```python
from build123d import *

# Parameters (mm, degrees)
PAD_DEPTH         = 18
PAD001_DEPTH      = 5
SKETCH002_W       = 13.704409
SKETCH002_H       = 6
POCKET_DEPTH      = 10.001
POCKET_DEPTH_BACK = -10.001
SKETCH003_R       = 6
PAD002_DEPTH      = 10
SKETCH004_R       = 1.5
POCKET001_DEPTH   = 10


with BuildPart() as part:
    # Sketch → Pad (new body)
    with BuildSketch(Plane.XY):
        with BuildLine():
            Line((-10, 0), (10, 0))
            Line((10, 0), (10, 8))
            Line((10, 8), (3.527972, 11.180071))
            ThreePointArc((3.527972, 11.180071), (0, 12), (-3.527972, 11.180071))
            Line((-3.527972, 11.180071), (-10, 8))
            Line((-10, 8), (-10, 0))
        make_face()
    extrude(amount=PAD_DEPTH)

    # Sketch001 → Pad001 (join)
    with BuildSketch(Plane.XY):
        with BuildLine():
            Line((-10, 0), (10, 0))
            Line((10, 0), (10, 10))
            ThreePointArc((10, 10), (0, 20), (-10, 10))
            Line((-10, 10), (-10, 0))
        make_face()
    extrude(amount=PAD001_DEPTH)

    # Sketch002 → Pocket (cut, two sides)
    with BuildSketch(Plane.YZ) as pocket_sk:
        with Locations((11.852204, 8)):
            Rectangle(SKETCH002_W, SKETCH002_H)
    extrude(amount=-POCKET_DEPTH, mode=Mode.SUBTRACT)
    extrude(pocket_sk.sketch, amount=-POCKET_DEPTH_BACK, mode=Mode.SUBTRACT)

    # Sketch003 (on Face4 of Pocket) → Pad002 (join)
    with BuildSketch(Plane(origin=(0, 0, 0), x_dir=(1, 0, 0), z_dir=(0, 0, -1))):
        with Locations((0, -10)):
            Circle(SKETCH003_R)
    extrude(amount=PAD002_DEPTH)

    # Sketch004 (on Face14 of Pad002) → Pocket001 (cut)
    with BuildSketch(Plane(origin=(0, 0, -10), x_dir=(1, 0, 0), z_dir=(0, 0, -1))):
        with Locations((0, -10)):
            Circle(SKETCH004_R)
    extrude(amount=-POCKET001_DEPTH, mode=Mode.SUBTRACT)


solid = part.part
```
Input: part model. Units: mm. Frame: model coordinates. A direction names the side the tool comes from. Round coordinates to 2 decimals unless told otherwise and drop trailing zeros. Loops run counter-clockwise (first coordinate to the right, second up) from the corner with the lowest first, then second, coordinate; pieces in that order, holes last. Notation, with made-up numbers: M 69.5,-20 L 86.5,-20 A26 cw 86.5,-4 Z; hole C 26.25,65 d6. An arc over 180 degrees is marked long. Answer in a Markdown table with one row per item. Add a question column.
1. Section C-C (z = 16). Output: boundary loops of the cut face in (x, y), and give its area (3 significant figures).
2. Section B-B (x = 0). Output: boundary loops of the cut face in (y, z).
3. Section A-A (y = 9.5). Output: boundary loops of the cut face in (x, z), and give its area (3 significant figures).
4. Set-up query: faces 4 (the face through (-0.78, 4.05, -4.93)), 5 (the face through (0, 12, 14)), 6 (the face through (6.809, 9.568, 14.451)). Return all of +Z, -Z, +X, -X, +Y, -Y with unobstructed straight access to the full face (end or side cutting, diameter ignored); none if empty.
5. Ray query, probe 1 along Y at (x, z) = (0, -7.5); probe 2 along X at (y, z) = (10, -2); probe 3 along Z at (x, y) = (-5, 5.75). Return the intervals inside material, ascending.
6. Mould query, pull axis Y, two halves, no side actions, for faces 1 (the face through (0, 8, 11)), 2 (the face through (0, 10, 0)), 3 (the face through (0, 5, 8)). Classes: released by +Y, released by -Y, zero draft, split by the parting line, or undercut.
7. Contact query for flat-ended pins moving along their axis: pin 1 (3 mm diameter, centred on y = 14, z = -4, fed in from -X); pin 2 (1.8 mm diameter, centred on x = -0.5, z = 8.5, fed in from +Y); pin 3 (3 mm diameter, centred on y = 13, z = -3.5, fed in from +X). Output: stop coordinate, or through.
8. Section D-D (y = 13.25). Output: boundary loops of the cut face in (x, z), and give its area (3 significant figures).
Values follow:
| question | item | result |
|---|---|---|
| 1 | outline | M -10,0 L 10,0 L 10,8 L 3.53,11.18 A8 ccw -3.53,11.18 L -10,8 Z |
| 1 | area | 207 mm^2 |
| 2 | outline | M 0,0 L 4,0 L 4,-10 L 8.5,-10 L 8.5,0 L 11.5,0 L 11.5,-10 L 16,-10 L 16,0 L 20,0 L 20,5 L 5,5 L 5,11 L 12,11 L 12,18 L 0,18 Z |
| 3 | outline | M -10,0 L -5.98,0 L -5.98,-10 L -1.41,-10 L -1.41,0 L 1.41,0 L 1.41,-10 L 5.98,-10 L 5.98,0 L 10,0 L 10,5 L -10,5 Z; M -6.95,11 L 6.95,11 L 6.95,18 L -6.95,18 Z |
| 3 | area | 289 mm^2 |
| 4 | face 4 | -Z |
| 4 | face 5 | +Z, +Y |
| 4 | face 6 | +Z, +X, +Y |
| 5 | probe 1 | 4 to 8.5, 11.5 to 16 |
| 5 | probe 2 | -6 to -1.5, 1.5 to 6 |
| 5 | probe 3 | 0 to 5, 11 to 18 |
| 6 | face 1 | zero draft |
| 6 | face 2 | undercut |
| 6 | face 3 | released by +Y |
| 7 | pin 1 | x = -5.45 |
| 7 | pin 2 | y = 5 |
| 7 | pin 3 | x = 5.81 |
| 8 | outline | M -9.46,0 L -5.04,0 L -5.04,-10 L 5.04,-10 L 5.04,0 L 9.46,0 L 9.46,5 L -9.46,5 Z |
| 8 | area | 195 mm^2 |
